Design review of the part built by this model. Coordinates are the model's own, in mm. A direction names the side the tool comes from. Coordinates: 2 decimals unless noted, no trailing zeros. Loops run counter-clockwise (first coordinate to the right, second up) from the corner with the lowest first, then second, coordinate; pieces in that order, holes last. Notation, with made-up numbers: (84.5, 54.5) -> (96.5, 54.5) arc R27 cw to (96.5, 80.5) -> close; hole circle Ø9 at (-40, -1). An arc over 180 degrees is marked (long way). Answer in a Markdown table with one row per item.
```python
from build123d import *

# Parameters (mm, degrees)
F1_DEPTH = 1.4
F0_R     = 2.25
F0_R_2   = 5
F2_DEPTH = 0.85
F3_W     = 52
F3_H     = 39.4
F3_W_2   = 49.4
F3_H_2   = 37
F4_DEPTH = 1.4
F6_R     = 3.1
F6_R_2   = 2.3
F7_DEPTH = 45
F8_R     = 5
F5_W     = 6.45
F5_H     = 1.1
F9_DEPTH = 0.55


with BuildPart() as f1:
    # F0 (on Front) → F1 (new body)
    with BuildSketch(Plane.XZ):
        Polygon((2.5, -14.9), (-2.5, -14.9), (-3.05, -14.9), (-3.05, -19.6), (3.05, -19.6), (3.05, -14.9), align=None)
    extrude(amount=-F1_DEPTH)

    # F0 (on Front) → F2 (join, symmetric)
    with BuildSketch(Plane.XZ):
        Polygon((-28.7, -22.5), (28.7, -22.5), (28.7, 22.5), (3.7, 22.5), (3.7, 19.8), (-3.7, 19.8), (-3.7, 22.5), (-28.7, 22.5), align=None)
        Polygon((-3.05, -14.9), (-2.5, -14.9), (2.5, -14.9), (3.05, -14.9), (3.05, -19.6), (-3.05, -19.6), align=None, mode=Mode.SUBTRACT)
        with BuildLine():
            add(Edge.make_bspline(
                [(-17.7, -2.85), (-14.3683195671, -2.85), (-16.0341597836, 1.425), (-17.7, 5.7), (-19.3658402164, 1.425), (-21.0316804329, -2.85), (-17.7, -2.85)],
                knots=[0, 0, 0, 2.0943951024, 2.0943951024, 4.1887902048, 4.1887902048, 6.2831853072, 6.2831853072, 6.2831853072], degree=2, weights=[1, 0.5, 1, 0.5, 1, 0.5, 1]))
        make_face(mode=Mode.SUBTRACT)
        with Locations((-9.05, -3.2)):
            Circle(F0_R, mode=Mode.SUBTRACT)
        with Locations((0, -1.1)):
            Circle(F0_R_2, mode=Mode.SUBTRACT)
        with Locations((9.05, -3.2)):
            Circle(F0_R, mode=Mode.SUBTRACT)
        with Locations((0, 9.15)):
            Circle(F0_R, mode=Mode.SUBTRACT)
    extrude(amount=F2_DEPTH, both=True)

    # F3 (on Front) → F4 (join)
    with BuildSketch(Plane.XZ):
        with Locations((0, 0.1)):
            Rectangle(F3_W, F3_H)
        Rectangle(F3_W_2, F3_H_2, mode=Mode.SUBTRACT)
    extrude(amount=-F4_DEPTH)

    # F6 (on face) → F7 (join)
    with BuildSketch(Plane(origin=(0, 0.85, 0), x_dir=(-1, 0, 0), z_dir=(0, 1, 0))):
        with Locations((-20.7, -10.4)):
            Circle(F6_R)
        with Locations((-20.7, -10.4)):
            Circle(F6_R_2, mode=Mode.SUBTRACT)
        with Locations((20.7, -10.4)):
            Circle(F6_R)
        with Locations((20.7, -10.4)):
            Circle(F6_R_2, mode=Mode.SUBTRACT)
    extrude(amount=F7_DEPTH)

    # F8
    f8_edges = [f1.edges().sort_by_distance(p)[0] for p in [
        (28.7, 0, -22.5),
        (-28.7, 0, -22.5),
    ]]
    fillet(f8_edges, radius=F8_R)

    # F5 (on face) → F9 (cut, symmetric)
    with BuildSketch(Plane(origin=(0, 1.4, 0), x_dir=(-1, 0, 0), z_dir=(0, 1, 0))):
        with Locations((-6.275, -19.05)):
            Rectangle(F5_W, F5_H)
        with Locations((6.275, -19.05)):
            Rectangle(F5_W, F5_H)
    extrude(amount=F9_DEPTH, both=True, mode=Mode.SUBTRACT)


solid = f1.part
```
(1) Take a section at A-A on z = 6. Give the boundary of the cut face in (x, y).
Evaluation:
| item | result |
|---|---|
| outline | (-28.7, -0.85) -> (28.7, -0.85) -> (28.7, 0.85) -> (26, 0.85) -> (26, 1.4) -> (24.7, 1.4) -> (24.7, 0.85) -> (-24.7, 0.85) -> (-24.7, 1.4) -> (-26, 1.4) -> (-26, 0.85) -> (-28.7, 0.85) -> close |
(2) For pin 1 (2.5 mm diameter, centred on x = -0.5, z = -16, fed in from +Y); pin 2 (0.6 mm diameter, centred on x = -1, y = 1, fed in from +Z); pin 3 (4 mm diameter, centred on x = -9.05, z = -3.2, fed in from +Y); pin 4 (1 mm diameter, centred on x = -7.5, z = 11, fed in from +Y), all flat-tipped, find the tip position at first contact; note any pin that passes through.
Evaluation:
| item | result |
|---|---|
| pin 1 | stops at y = 1.4 |
| pin 2 | stops at z = 19.8 |
| pin 3 | passes through |
| pin 4 | stops at y = 0.85 |
(3) To check wall thickness, follow probe 1 along Z at (x, y) = (20.7, 24); probe 2 along Y at (x, z) = (-11, 3); probe 3 along X at (y, z) = (8, -12). State the ranges of each line that lie inside material, in increasing order.
Evaluation:
| item | result |
|---|---|
| probe 1 | z = -13.5 to -12.7, -8.1 to -7.3 |
| probe 2 | y = -0.85 to 0.85 |
| probe 3 | x = -23.36 to -22.35, -19.05 to -18.04, 18.04 to 19.05, 22.35 to 23.36 |
(4) Draft analysis for pull direction Z (two halves, no side actions). For faces 1 (the flat face through (0, 1.4, 19)), 2 (the flat face through (16, 0, 22.5)), 3 (the flat face through (0, 0, -17)), 4 (the flat face through (0, 0, -22.5)), state which applies: pulls with the +Z half, pulls with the -Z half, needs draft (parallel to the pull), parting line crosses it, or undercut.
Evaluation:
| item | result |
|---|---|
| face 1 | needs draft |
| face 2 | pulls with the +Z half |
| face 3 | undercut |
| face 4 | pulls with the -Z half |
(5) Tool access review of faces 5 (the flat face through (-21, 0.85, -10)), 6 (the flat face through (28.7, 0, 2)): name each direction out of +Z, -Z, +X, -X, +Y, -Y from which nothing blocks a thin tool from reaching the whole face with its end or side.
Evaluation:
| item | result |
|---|---|
| face 5 | +Y |
| face 6 | +Z, -Z, +X, +Y, -Y |
(6) Take a section at D-D on z = -10.4. Give the boundary of the cut face in (x, y).
Evaluation:
| item | result |
|---|---|
| outline | (-28.7, -0.85) -> (28.7, -0.85) -> (28.7, 0.85) -> (26, 0.85) -> (26, 1.4) -> (24.7, 1.4) -> (24.7, 0.85) -> (23.8, 0.85) -> (23.8, 45.85) -> (23, 45.85) -> (23, 0.85) -> (18.4, 0.85) -> (18.4, 45.85) -> (17.6, 45.85) -> (17.6, 0.85) -> (-17.6, 0.85) -> (-17.6, 45.85) -> (-18.4, 45.85) -> (-18.4, 0.85) -> (-23, 0.85) -> (-23, 45.85) -> (-23.8, 45.85) -> (-23.8, 0.85) -> (-24.7, 0.85) -> (-24.7, 1.4) -> (-26, 1.4) -> (-26, 0.85) -> (-28.7, 0.85) -> close |
(7) Take a section at C-C on y = 31. Give the boundary of the cut face in (x, z), and give its area (3 significant figures).
Evaluation:
| item | result |
|---|---|
| outline | circle Ø6.2 at (-20.7, -10.4); circle Ø6.2 at (20.7, -10.4); hole circle Ø4.6 at (-20.7, -10.4); hole circle Ø4.6 at (20.7, -10.4) |
| area | 27.1 mm² |
(8) Take a section at B-B on x = 20.7. Give the boundary of the cut face in (y, z), and give its area (3 significant figures).
Evaluation:
| item | result |
|---|---|
| outline | (-0.85, -22.5) -> (0.85, -22.5) -> (0.85, -19.6) -> (1.4, -19.6) -> (1.4, -18.5) -> (0.85, -18.5) -> (0.85, -13.5) -> (45.85, -13.5) -> (45.85, -12.7) -> (0.85, -12.7) -> (0.85, -8.1) -> (45.85, -8.1) -> (45.85, -7.3) -> (0.85, -7.3) -> (0.85, 18.5) -> (1.4, 18.5) -> (1.4, 19.8) -> (0.85, 19.8) -> (0.85, 22.5) -> (-0.85, 22.5) -> close |
| area | 150 mm² |
